Here's how the part is built. I have some questions about the finished solid (model axes, mm). Face numbers are marked on the shaded views. A direction names the side the tool comes from. Round coordinates to 2 decimals unless told otherwise and drop trailing zeros. Write each loop counter-clockwise with the first axis right and the second up, starting at its lowest first coordinate (ties: lowest second). Pieces come first, ordered by that corner, then holes. Notation, with made-up numbers: (34, -11) -> (56, -11) arc R12 cw to (56, 2) -> close; hole circle Ø5 at (59, 14.5). An arc over 180 degrees is marked (long way). Answer as CSV lines item,"result".
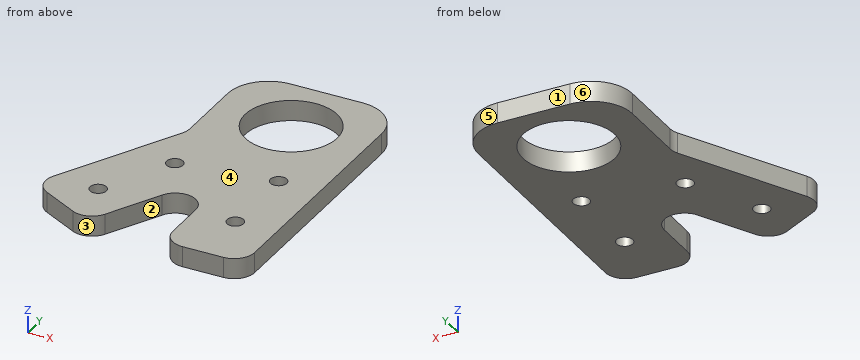
Autodesk Inventor part; units mm, degrees
ref_plane "YZ Plane" through (0, 0, 0) normal (1, 0, 0) x (0, 1, 0)
ref_plane "XZ Plane" through (0, 0, 0) normal (0, 1, 0) x (-1, 0, 0)
ref_plane "XY Plane" through (0, 0, 0) normal (0, 0, 1) x (1, 0, 0)
sketch "Sketch1" plane through (0, 0, 0) normal (0, 0, 1) x (1, 0, 0)
  line L0 (-12.7, 0) -> (12.7, 0) construction
  line L1 (12.7, 0) -> (12.7, -57.15)
  line L2 (12.7, -57.15) -> (-12.7, -57.15)
  line L3 (-12.7, -57.15) -> (-12.7, 0) construction
  line L4 (-35.1269, 0) -> (-12.7, -11.9246) construction
  line L5 (-12.7, -11.9246) -> (-36.5492, -56.7783)
  line L6 (-36.5492, -56.7783) -> (-58.976, -44.8537)
  line L7 (-58.976, -44.8537) -> (-35.1269, 0)
  line L8 (-23.9134, -5.9623) -> (-47.7626, -50.816) construction
  line L9 (-35.1269, 0) -> (12.7, 0)
  line L10 (-12.7, -11.9246) -> (-12.7, -57.15)
  point P0 (0, 0)
  point P1 (0, 0)
  point P2 (-29.8757, -17.1757)
  point P3 (-41.8003, -39.6026)
  point P4 (0, -12.7)
  point P5 (0, -38.1)
  dimension "d0" = 25.4
  dimension "d1" = 25.4
  dimension "d2" = 28
  dimension "d3" = 50.8
  dimension "d4" = 25.4
  dimension "d5" = 12.7
  dimension "d6" = 25.4
  dimension "d7" = 12.7
  dimension "d8" = 57.15
extrude "Extrusion1" add sketch "Sketch1" against normal blind 6.35
hole "Hole1" at (-29.8757, -17.1757, 0) at (-41.8003, -39.6026, 0) at (0, -12.7, 0) at (0, -38.1, 0) direction (0, 0, -1) diameter 5.1054 end through all
sketch "Sketch2" plane through (0, 0, 0) normal (0, 0, 1) x (1, 0, 0)
  circle A0 centre (0, -12.7) radius 2.5527 construction
  circle A1 centre (-29.8757, -17.1757) radius 2.5527 construction
  circle A2 centre (-41.8003, -39.6026) radius 2.5527 construction
  circle A3 centre (0, -38.1) radius 2.5527 construction
  line L0 (-12.7, -57.15) -> (12.7, -57.15) construction
  line L1 (12.7, -57.15) -> (12.7, 0) construction
  line L2 (12.7, 0) -> (-35.1269, 0)
  line L3 (-35.1269, 0) -> (-58.976, -44.8537) construction
  line L4 (-58.976, -44.8537) -> (-36.5492, -56.7783) construction
  line L5 (-36.5492, -56.7783) -> (-12.7, -11.9246) construction
  line L6 (-12.7, -11.9246) -> (-12.7, -57.15) construction
  circle A4 centre (0, -12.7) radius 2.5527 construction
  circle A5 centre (-29.8757, -17.1757) radius 2.5527 construction
  circle A6 centre (-41.8003, -39.6026) radius 2.5527 construction
  circle A7 centre (0, -38.1) radius 2.5527 construction
  line L7 (12.7, 0) -> (12.7, -57.15) construction
  line L8 (12.7, -57.15) -> (-12.7, -57.15) construction
  line L9 (-12.7, -57.15) -> (-12.7, -11.9246) construction
  line L10 (-36.5492, -56.7783) -> (-58.976, -44.8537) construction
  line L11 (-58.976, -44.8537) -> (-35.1269, 0) construction
  line L12 (-35.1269, 0) -> (12.7, 0) construction
  circle A8 centre (-11.2134, 15.875) radius 14.2875 construction
  line L13 (12.7, 0) -> (-35.1269, 0) construction
  line L14 (-35.1269, 0) -> (-58.976, -44.8537) construction
  circle A9 centre (0, -12.7) radius 2.5527 construction
  circle A10 centre (-29.8757, -17.1757) radius 2.5527 construction
  circle A11 centre (-41.8003, -39.6026) radius 2.5527 construction
  circle A12 centre (0, -38.1) radius 2.5527 construction
  line L15 (12.7, 0) -> (12.7, -57.15) construction
  line L16 (12.7, -57.15) -> (-12.7, -57.15) construction
  line L17 (-12.7, -57.15) -> (-12.7, -11.9246) construction
  line L18 (-36.5492, -56.7783) -> (-58.976, -44.8537) construction
  line L19 (-58.976, -44.8537) -> (-35.1269, 0) construction
  line L20 (-35.1269, 0) -> (12.7, 0) construction
  line L21 (-35.1269, 0) -> (12.7, 0) construction
  line L22 (12.7, 0) -> (12.7, 36.5125)
  line L23 (12.7, 36.5125) -> (-35.1269, 36.5125)
  line L24 (-35.1269, 36.5125) -> (-35.1269, 0)
  line L25 (-12.7, -11.9246) -> (-36.5492, -56.7783)
  line L26 (-12.7, -11.9246) -> (-36.5492, -56.7783)
  point P0 (0, 0)
  point P1 (-11.2134, 0)
  point P2 (-11.2134, 0)
  point P3 (-11.2134, 30.1625)
  point P4 (-11.2134, 36.5125)
  dimension "d19" = 28.575
  dimension "d20" = 15.875
  dimension "d21" = 6.35
extrude "Extrusion2" add sketch "Sketch2" against normal up to surface (6.35 mm away)
hole "Hole2" at (-11.2134, 15.875, 0) direction (0, 0, -1) diameter 28.575 end through all
fillet "Fillet1" radius 6.35 6 edges at (12.7, -57.15, -3.175) (-12.7, -57.15, -3.175) (-12.7, -11.9246, -3.175) (-36.5492, -56.7783, -3.175) (-58.976, -44.8537, -3.175) (-35.1269, 0, -3.175)
fillet "Fillet2" radius 12.7 2 edges at (-35.1269, 36.5125, -3.175) (12.7, 36.5125, -3.175)
properties part number "CL4-010" material "Aluminum 6061"
Item 1: Suppose I cut it at A-A, the plane y = 3. List the corners of the cut face in (x, z) for me.
Results found:
outline,"(-35.13, -6.35) -> (-17.41, -6.35) -> (-17.41, 0) -> (-35.13, 0) -> close; (-5.02, -6.35) -> (12.7, -6.35) -> (12.7, 0) -> (-5.02, 0) -> close"
Item 2: Will these pins go through, and if not, where does the flat tip stop? pin 1 (1.9 mm diameter, centred on y = 18, z = -3.5, fed in from -X); pin 2 (8 mm diameter, centred on x = -29.88, y = -17.18, fed in from -Z).
Results found:
pin 1,"stops at x = -35.13"
pin 2,"stops at z = -6.35"
Item 3: Suppose I cut it at B-B, the plane z = -4. State how many separate pieces and enclosed holes the cut face has, then the cut area to 3 significant figures.
Results found:
separate pieces,"1"
enclosed holes,"5"
area,"3,900 mm²"
Item 4: If we mould it in two halves opening along X, with no side actions, what happens to the marked faces 3, 4, 5 and 6? For each: pulls with the +X half, pulls with the -X half, needs draft (parallel to the pull), parting line crosses it, or undercut.
Results found:
face 3,"undercut"
face 4,"needs draft"
face 5,"pulls with the +X half"
face 6,"pulls with the -X half"
Item 5: I need wall thicknesses on L1, parallel to X at y = -36, z = -1.25; L2, parallel to Y at x = 0, z = -4.75; L3, parallel to Y at x = 2, z = -2.75. Which ranges of each line are inside material? Lowest first, please.
Results found:
L1,"x = -54.27 to -25.5, -12.85 to -1.45, 1.45 to 12.7"
L2,"y = -57.15 to -40.65, -35.55 to -15.25, -10.15 to 7.02, 24.73 to 36.51"
L3,"y = -57.15 to -39.69, -36.51 to -14.29, -11.11 to 10.44, 21.31 to 36.35"
Item 6: For the marked faces 1 and 2, which set-ups out of +Z, -Z, +X, -X, +Y, -Y let a thin tool reach every point of the face, with its end or its side?
Results found:
face 1,"+Z, -Z, +X, -X, +Y"
face 2,"+Z, -Z, -Y"
Item 7: Suppose I cut it at D-D, the plane x = -51. List the corners of the cut face in (y, z) for me.
Results found:
outline,"(-49.09, -6.35) -> (-29.85, -6.35) -> (-29.85, 0) -> (-49.09, 0) -> close"
Item 8: Suppose I cut it at C-C, the plane y = -12.7. List the corners of the cut face in (x, z) for me.
Results found:
outline,"(-41.88, -6.35) -> (-2.55, -6.35) -> (-2.55, 0) -> (-41.88, 0) -> close; (2.55, -6.35) -> (12.7, -6.35) -> (12.7, 0) -> (2.55, 0) -> close"
